Work out the finished part from the listing and answer in its coordinate system (mm). Round coordinates to 2 decimals unless told otherwise and drop trailing zeros. Write each loop counter-clockwise with the first axis right and the second up, starting at its lowest first coordinate (ties: lowest second). Pieces come first, ordered by that corner, then holes. Notation, with made-up numbers: (18, 84.25) - (47, 84.25) arc R24 cw to (47, 113.25) - close; hole circle Ø4 at (-15.75, 71.5). An arc over 180 degrees is marked (long way). Answer as a JSON object with one key per item and string values.
```python
from build123d import *

# Parameters (mm, degrees)
SKETCH2_R           = 381
BOSS_EXTRUDE1_DEPTH = 355.6
SKETCH3_R           = 279.4
CUT_EXTRUDE1_DEPTH  = 646.579863379
FILLET3_R           = 25.4
FILLET4_R           = 25.4
SCALE1_SCALE        = 0.15


with BuildPart() as part:
    # Sketch2 → Boss-Extrude1 (new body)
    with BuildSketch(Plane.XY):
        Circle(SKETCH2_R)
    extrude(amount=BOSS_EXTRUDE1_DEPTH)

    # Sketch3 → Cut-Extrude1 (cut, through all)
    with BuildSketch(Plane.XY.offset(355.6)):
        Circle(SKETCH3_R)
    extrude(amount=-CUT_EXTRUDE1_DEPTH, mode=Mode.SUBTRACT)

    # Fillet3
    fillet3_edges = [part.edges().sort_by_distance(p)[0] for p in [
        (-381, 0, 0),
        (-381, 0, 355.6),
    ]]
    fillet(fillet3_edges, radius=FILLET3_R)

    # Fillet4
    fillet4_edges = [part.edges().sort_by_distance(p)[0] for p in [
        (-279.4, 0, 0),
        (-279.4, 0, 355.6),
    ]]
    fillet(fillet4_edges, radius=FILLET4_R)


with BuildPart() as part_1:
    # Scale1: scaled about (0, 0, 177.8)
    add(part.part.scale(SCALE1_SCALE).moved(Location((0, 0, 151.13))))


solid = part_1.part
```
Item 1: A cutting plane is placed at A-A (x = 0). Write down the section's boundary in (y, z), and give its area (3 significant figures).
Results found:
{"outline": "(-57.15, 154.94) arc R3.81 ccw to (-53.34, 151.13) - (-45.72, 151.13) arc R3.81 ccw to (-41.91, 154.94) - (-41.91, 200.66) arc R3.81 ccw to (-45.72, 204.47) - (-53.34, 204.47) arc R3.81 ccw to (-57.15, 200.66) - close; (41.91, 154.94) arc R3.81 ccw to (45.72, 151.13) - (53.34, 151.13) arc R3.81 ccw to (57.15, 154.94) - (57.15, 200.66) arc R3.81 ccw to (53.34, 204.47) - (45.72, 204.47) arc R3.81 ccw to (41.91, 200.66) - close", "area": "1,600 mm²"}
Item 2: Consider line 1 along Y through (x, z) = (0, 183); line 2 along X through (y, z) = (-20.5, 198.5). Determine where each line is inside the solid, lowest interval first.
Results found:
{"line 1": "-57.15 to -41.91, 41.91 to 57.15", "line 2": "-53.35 to -36.55, 36.55 to 53.35"}
Item 3: Determine the mould class of faces 1 (the flat face through (39.3, 24, 151.13)), 2 (the cylindrical face through (-57.095, 2.513, 177.48)), 3 (the cylindrical face through (-5.456, 41.553, 178.12)) for opening direction Y: pulls with the +Y half, pulls with the -Y half, needs draft (parallel to the pull), parting line crosses it, or undercut.
Results found:
{"face 1": "needs draft", "face 2": "parting line crosses it", "face 3": "undercut"}
Item 4: A cutting plane is placed at C-C (z = 176). Write down the section's boundary in (x, y), and give its area (3 significant figures).
Results found:
{"outline": "circle Ø114.3 at (0, 0); hole circle Ø83.82 at (0, 0)", "area": "4,740 mm²"}
Item 5: Each of these flat-tipped pins is pushed along its axis until it touches: P1, Ø4, axis at y = 43, z = 178, coming from the -X side; P2, Ø10, axis at x = -10.5, z = 187, coming from the -Y side; P3, Ø4, axis at y = 39, z = 185.5, coming from the -X side. Where does it stop, or does it pass through?
Results found:
{"P1": "x = -39.81", "P2": "y = -56.88", "P3": "x = -43.56"}
